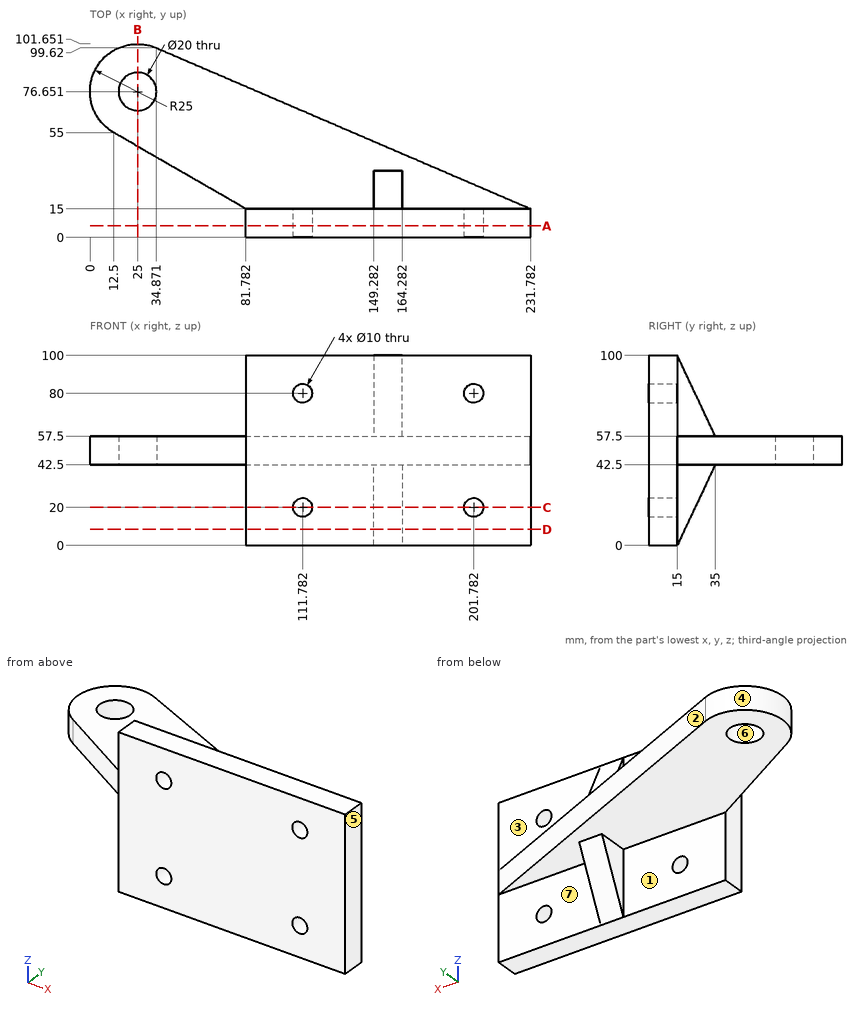
The drawing under review shows one solid part. Ordinate dimensions are in mm from its lowest x, y, z. A direction names the side the tool comes from. Coordinates: 2 decimals unless noted, no trailing zeros. Loops run counter-clockwise (first coordinate to the right, second up) from the corner with the lowest first, then second, coordinate; pieces in that order, holes last. Notation, with made-up numbers: (35, 80) -> (90, 80) arc R15 ccw to (90, 86) -> close; hole circle Ø5 at (-14.75, 50). An arc over 180 degrees is marked (long way). Answer as a JSON object with one key per item and string values.
Q1. Take a section at D-D on z = 8.5. Give the boundary of the cut face in (x, y), plus the area to 3 significant figures.
Answer block:
{"outline": "(81.78, 0) -> (231.78, 0) -> (231.78, 15) -> (164.28, 15) -> (164.28, 19) -> (149.28, 19) -> (149.28, 15) -> (81.78, 15) -> close", "area": "2,310 mm^2"}
Q2. The part is to be moulded in two halves that separate along X. For the marked faces 4, 5, 6 and 7, say which applies: +X half, -X half, draft (parallel to the pull), parting line (faces both ways), or undercut.
Answer block:
{"face 4": "parting line", "face 5": "+X half", "face 6": "undercut", "face 7": "draft"}
Q3. Tool access review of the marked faces 1, 2 and 3: name each direction out of +Z, -Z, +X, -X, +Y, -Y from which nothing blocks a thin tool from reaching the whole face with its end or side.
Answer block:
{"face 1": "-Z, -X, +Y", "face 2": "+Z, -Z, +X, +Y", "face 3": "+Z, +X, +Y"}
Q4. Take a section at A-A on y = 6. Give the boundary of the cut face in (x, z).
Answer block:
{"outline": "(81.78, 0) -> (231.78, 0) -> (231.78, 100) -> (81.78, 100) -> close; hole circle Ø10 at (111.78, 20); hole circle Ø10 at (111.78, 80); hole circle Ø10 at (201.78, 20); hole circle Ø10 at (201.78, 80)"}
Q5. Clearance check with flat-ended pins moving along their axes: pin 1 Ø22 at (y, z) = (29, 80) entering from -X; pin 2 Ø4.5 at (y, z) = (8.5, 51) entering from -X; pin 3 Ø21 at (x, z) = (207, 88.5) entering from +Y. State where each tip first meets the part, or that it passes through.
Answer block:
{"pin 1": "stops at x = 149.28", "pin 2": "stops at x = 81.78", "pin 3": "stops at y = 15"}
Q6. Take a section at B-B on x = 25. Give the boundary of the cut face in (y, z).
Answer block:
{"outline": "(47.78, 42.5) -> (66.65, 42.5) -> (66.65, 57.5) -> (47.78, 57.5) -> close; (86.65, 42.5) -> (101.65, 42.5) -> (101.65, 57.5) -> (86.65, 57.5) -> close"}
Q7. Take a section at C-C on z = 20. Give the boundary of the cut face in (x, y).
Answer block:
{"outline": "(81.78, 0) -> (106.78, 0) -> (106.78, 15) -> (81.78, 15) -> close; (116.78, 0) -> (196.78, 0) -> (196.78, 15) -> (164.28, 15) -> (164.28, 24.41) -> (149.28, 24.41) -> (149.28, 15) -> (116.78, 15) -> close; (206.78, 0) -> (231.78, 0) -> (231.78, 15) -> (206.78, 15) -> close"}
Q8. To check wall thickness, follow L1, parallel to X at y = 7, z = 20; L2, parallel to Y at x = 179, z = 14; L3, parallel to Z at x = 126, y = 26.5. State the ranges of each line that lie inside material, in increasing order.
Answer block:
{"L1": "x = 81.78 to 106.78, 116.78 to 196.78, 206.78 to 231.78", "L2": "y = 0 to 15", "L3": "z = 42.5 to 57.5"}
